Can you work these out from the model? Positions are in its coordinate system, mm. Give positions to 0.01 mm unless a question says otherwise; leave off trailing zeros. Order: outer loops, then holes, each group sorted by start corner. A loop starts at its lowest first (then second) coordinate and runs counter-clockwise, first axis right, second up. Notation, with made-up numbers: M 24,48.5 L 73,48.5 A29 ccw 73,78.5 Z; hole C 30.5,44.5 d2. An arc over 180 degrees is marked long. Answer as a JSON object with one key per item and string values.
```python
from build123d import *

# Parameters (mm, degrees)
BOSS_EXTRUDE1_DEPTH = 15


with BuildPart() as part:
    # Sketch1 → Boss-Extrude1 (new body)
    with BuildSketch(Plane(origin=(0, 0, 0), x_dir=(1, 0, 0), z_dir=(0, 1, 0))):
        with BuildLine():
            ThreePointArc((-659.025122037, 412.448905192), (-659.689338477, 412.586057046), (-660.366005428, 412.632056457))
            Line((-660.366005428, 412.632056457), (-864.195118688, 412.632056457))
            ThreePointArc((-864.195118688, 412.632056457), (-865.324084301, 412.502932831), (-866.39473946, 412.122231116))
            Line((-866.39473946, 412.122231116), (-894.575915261, 398.316999834))
            ThreePointArc((-894.575915261, 398.316999834), (-909.423967253, 405.375573292), (-899.195089964, 418.246366617))
            Line((-899.195089964, 418.246366617), (-595.213920413, 418.24431837))
            ThreePointArc((-595.213920413, 418.24431837), (-594.262691586, 418.201142157), (-593.319285704, 418.071968602))
            Line((-593.319285704, 418.071968602), (-479.651763212, 397.219361415))
            ThreePointArc((-479.651763212, 397.219361415), (-466.351873551, 376.983335948), (-487.166106805, 364.607897137))
            Line((-487.166106805, 364.607897137), (-659.025122037, 412.448905192))
        make_face()
        with BuildLine():
            Line((-658.891051676, 412.930525483), (-487.045817139, 365.093353609))
            ThreePointArc((-487.045817139, 365.093353609), (-466.835293219, 377.176572267), (-479.911630321, 396.759188493))
            Line((-479.911630321, 396.759188493), (-593.409278239, 417.581166717))
            ThreePointArc((-593.409278239, 417.581166717), (-594.307856674, 417.704206285), (-595.213886711, 417.745334257))
            Line((-595.213886711, 417.745334257), (-899.19505992, 417.746358527))
            ThreePointArc((-899.19505992, 417.746358527), (-908.936889556, 405.488468327), (-894.795900883, 398.766001802))
            Line((-894.795900883, 398.766001802), (-866.61470183, 412.571185618))
            ThreePointArc((-866.61470183, 412.571185618), (-865.436984962, 412.989954476), (-864.195127301, 413.131989419))
            Line((-864.195127301, 413.131989419), (-660.366014041, 413.131989419))
            ThreePointArc((-660.366014041, 413.131989419), (-659.621685121, 413.081391266), (-658.891051676, 412.930525483))
        make_face(mode=Mode.SUBTRACT)
    extrude(amount=BOSS_EXTRUDE1_DEPTH)


solid = part.part
```
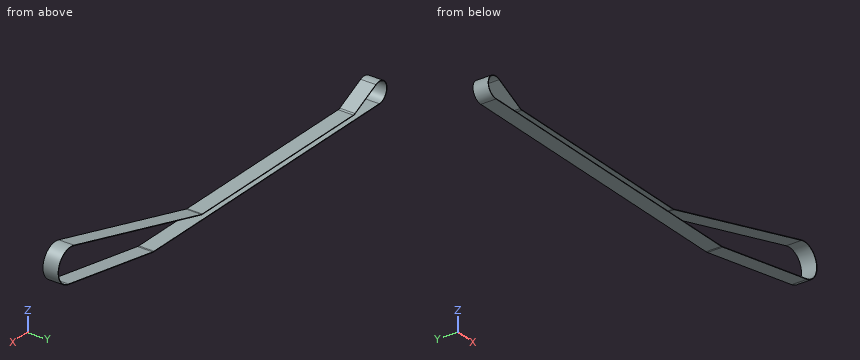
1) I want a section at B-B on z = -402.5. Write out the boundary of the cut face in (x, y), and give its area (3 significant figures).
Results found:
{"outline": "M -908.29,0 L -907.71,0 L -907.71,15 L -908.29,15 Z; M -887.17,0 L -886.04,0 L -886.04,15 L -887.17,15 Z; M -623.29,0 L -621.42,0 L -621.42,15 L -623.29,15 Z; M -511.2,0 L -508.44,0 L -508.44,15 L -511.2,15 Z", "area": "95.3 mm²"}
2) I want a section at C-C on x = -881. Write out the boundary of the cut face in (y, z).
Results found:
{"outline": "M 0,-418.25 L 15,-418.25 L 15,-417.75 L 0,-417.75 Z; M 0,-405.52 L 15,-405.52 L 15,-404.97 L 0,-404.97 Z"}
3) I need wall thicknesses on L1, parallel to Z at x = -683, y = 11; L2, parallel to Z at x = -580, y = 11.75. Which ranges of each line are inside material? Lowest first, please.
Results found:
{"L1": "z = -418.24 to -417.75, -413.13 to -412.63", "L2": "z = -415.63 to -415.12, -390.97 to -390.45"}
4) I want a section at D-D on z = -386. Write out the boundary of the cut face in (x, y).
Results found:
{"outline": "M -564.01,0 L -562.15,0 L -562.15,15 L -564.01,15 Z; M -467.31,0 L -466.77,0 L -466.77,15 L -467.31,15 Z"}
5) I'm going to push flat-ended pins straight in: pin 1 Ø1 at (y, z) = (6.5, -391.5) entering from +X; pin 2 Ø23 at (x, z) = (-899.2, -407.75) entering from +Y; pin 3 Ø4 at (x, y) = (-603, 3) entering from +Z. Where does each tip first touch, or does it pass through?
Results found:
{"pin 1": "stops at x = -469.43", "pin 2": "stops at y = 15", "pin 3": "stops at z = -396.3"}
6) I want a section at A-A on y = 6. Write out the boundary of the cut face in (x, z), and give its area (3 significant figures).
Results found:
{"outline": "M -899.2,-418.25 L -595.21,-418.24 A10.5 ccw -593.32,-418.07 L -479.65,-397.22 A16.75 ccw long -487.17,-364.61 L -659.03,-412.45 A5 cw -660.37,-412.63 L -864.2,-412.63 A5 cw -866.39,-412.12 L -894.58,-398.32 A10.5 ccw long Z; hole M -899.2,-417.75 L -595.21,-417.75 A10 ccw -593.41,-417.58 L -479.91,-396.76 A16.25 ccw long -487.05,-365.09 L -658.89,-412.93 A5.5 cw -660.37,-413.13 L -864.2,-413.13 A5.5 cw -866.61,-412.57 L -894.8,-398.77 A10 ccw long Z", "area": "465 mm²"}
